The listing builds one solid part. Answer for the finished solid, in the listing's coordinates (mm). A direction names the side the tool comes from. Round coordinates to 2 decimals unless told otherwise and drop trailing zeros. Write each loop counter-clockwise with the first axis right and the second up, starting at its lowest first coordinate (ties: lowest second). Pieces come first, ordered by that corner, then holes. Notation, with made-up numbers: (42.5, -26.5) - (71.5, -26.5) arc R34 ccw to (71.5, 12.5) - close; hole circle Ø1 at (-31.5, 7.25). An arc over 180 degrees is marked (long way). Return JSON: item names as keys, results as strings. Group by question number.
(1) Determine the mould class of faces 3 (the flat face through (6.904, -4, 4)), 4 (the flat face through (7, -4, -2)), 5 (the cylindrical face through (3.54, -10.74, -2.38)) for opening direction Y: +Y half, -Y half, draft (parallel to the pull), parting line (faces both ways), or undercut.
(2) Which of the six approach directions +Z, -Z, +X, -X, +Y, -Y give full straight-line access (tool end or side, diameter ignored) to faces 1 (the flat face through (0, -4, 2)), 2 (the flat face through (0.096, -4, -4))?
(3) Each of these flat-tipped pins is pushed along its axis until it touches: pin 1 (1 mm diameter, centred on y = -7, z = -2.5, fed in from +X); pin 2 (2 mm diameter, centred on x = 3.5, y = -1.5, fed in from -Z). Where does it stop, or does it pass through?
(4) Find the intervals of material crossed by line 1 along Y through (x, z) = (5, 0); line 2 along Y through (x, z) = (6.95, 0); line 3 along X through (y, z) = (-1, -7.5), in increasing order. Write a range as [from, to].
(5) Section C-C, the plane x = 5 is taken. Write down the section's boundary in (y, z).
```python
from build123d import *


with BuildPart() as part:
    # Sketch1 → Revolve1 (revolve)
    with BuildSketch(Plane(origin=(0, 0, 0), x_dir=(-1, 0, 0), z_dir=(0, 0, -1)), mode=Mode.PRIVATE) as revolve1_sk:
        with BuildLine():
            Line((-6.7, 4), (-0.3, 4))
            ThreePointArc((-0.3, 4), (-0.087867966, 4.087867966), (0, 4.3))
            Line((0, 4.3), (0, 5.2629))
            Line((0, 5.2629), (-0.0956, 5.2629))
            Line((-0.0956, 5.2629), (-0.0956, 9.6056))
            Line((-0.0956, 9.6056), (0, 9.6056))
            Line((0, 9.6056), (0, 10.7))
            ThreePointArc((0, 10.7), (-0.087867966, 10.912132034), (-0.3, 11))
            Line((-0.3, 11), (-6.7, 11))
            ThreePointArc((-6.7, 11), (-6.912132034, 10.912132034), (-7, 10.7))
            Line((-7, 10.7), (-7, 9.6056))
            Line((-7, 9.6056), (-6.9044, 9.6056))
            Line((-6.9044, 9.6056), (-6.9044, 5.2629))
            Line((-6.9044, 5.2629), (-7, 5.2629))
            Line((-7, 5.2629), (-7, 4.3))
            ThreePointArc((-7, 4.3), (-6.912132034, 4.087867966), (-6.7, 4))
        make_face()
    revolve(revolve1_sk.sketch.rotate(Axis((7.003537608, 0, 0), (-1, 0, 0)), 270), axis=Axis((7.003537608, 0, 0), (-1, 0, 0)))


solid = part.part
```
Working result:
{
 "1": {"face 3": "undercut", "face 4": "draft", "face 5": "parting line"},
 "2": {"face 1": "+Z, -Z, -X, +Y, -Y", "face 2": "-X"},
 "3": {"pin 1": "stops at x = 6.9", "pin 2": "stops at z = -10.99"},
 "4": {"line 1": "y = [-11, -4], [4, 11]", "line 2": "y = [-10.87, -9.61], [-5.26, -4.13], [4.13, 5.26], [9.61, 10.87]", "line 3": "x = [0.1, 6.9]"},
 "5": {"outline": "circle Ø22 at (0, 0); hole circle Ø8 at (0, 0)"}
}
